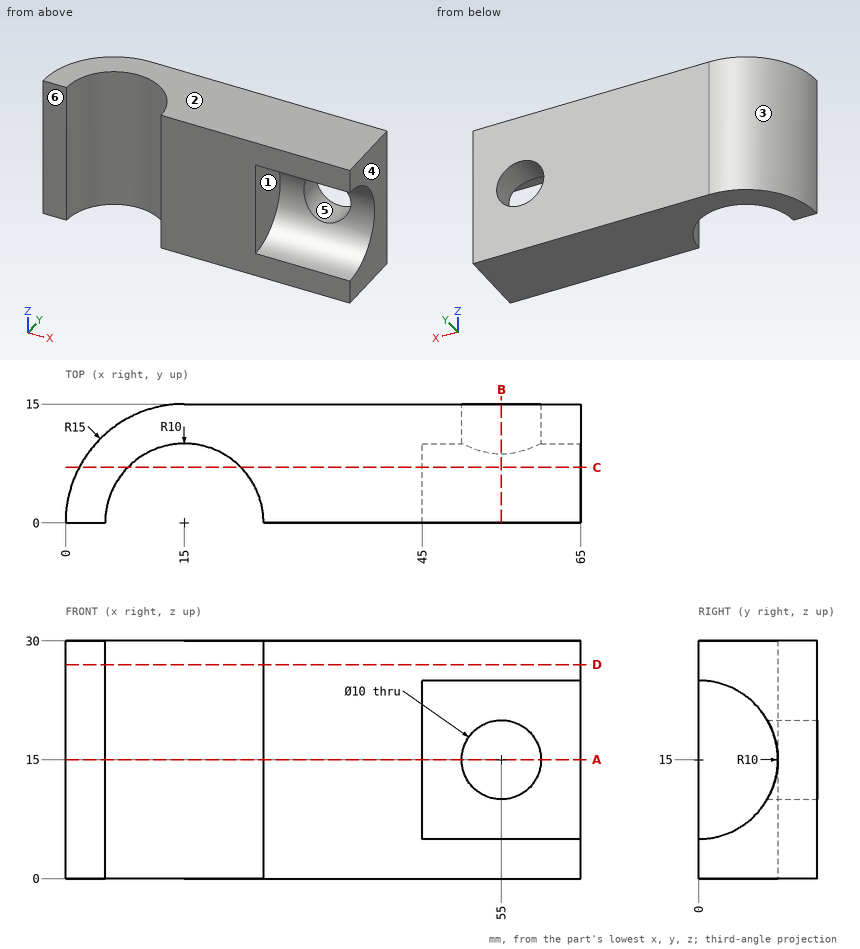
Could you check a few things on this drawing? It's one solid part, dimensions in mm from its lowest x, y, z. A direction names the side the tool comes from. Coordinates: 2 decimals unless noted, no trailing zeros. Order: outer loops, then holes, each group sorted by start corner. A loop starts at its lowest first (then second) coordinate and runs counter-clockwise, first axis right, second up.
1) Imagine slicing it at B-B on x = 55. List the corners of the cut face in (y, z) for me.
2) Imagine slicing it at D-D on z = 27. List the corners of the cut face in (x, y) for me, and give its area (3 significant figures).
3) We'd pull the mould along X, two halves only. Please class the marked faces 3, 4, 5 and 6: +X half, -X half, draft (parallel to the pull), parting line (faces both ways), or undercut.
4) Will these pins go through, and if not, where does the flat tip stop? pin 1 (5 mm diameter, centred on y = 5, z = 18.5, fed in from +X); pin 2 (1 mm diameter, centred on y = 11, z = 6, fed in from -X).
5) Imagine slicing it at A-A on z = 15. List the corners of the cut face in (x, y) for me.
6) Imagine slicing it at C-C on y = 7. List the corners of the cut face in (x, z) for me, and give its area (3 significant figures).
7) Which directions (+Z, -Z, +X, -X, +Y, -Y) give clear straight access to the entire face, cutting with the end or side of a thin tool? Please do the marked faces 1 and 2.
8) I need wall thicknesses on line 1 (Z direction, x = 55, y = 12.75); line 2 (X direction, y = 1, z = 27.5); line 3 (Z direction, x = 56, y = 1). Which ranges of each line are inside material? Lowest first, please.
Response values:
1. outline: (0, 0) - (15, 0) - (15, 10) - (8.66, 10) arc R10 cw to (0, 5) - close; (0, 25) arc R10 cw to (8.66, 20) - (15, 20) - (15, 30) - (0, 30) - close
2. outline: (0, 0) - (5, 0) arc R10 cw to (25, 0) - (65, 0) - (65, 15) - (15, 15) arc R15 ccw to start
2. area: 770 mm2
3. face 3: -X half
3. face 4: +X half
3. face 5: undercut
3. face 6: draft
4. pin 1: stops at x = 45
4. pin 2: stops at x = 4.29
5. outline: (0, 0) - (5, 0) arc R10 cw to (25, 0) - (45, 0) - (45, 10) - (50, 10) - (50, 15) - (15, 15) arc R15 ccw to start; (60, 10) - (65, 10) - (65, 15) - (60, 15) - close
6. outline: (1.73, 0) - (7.86, 0) - (7.86, 30) - (1.73, 30) - close; (22.14, 0) - (65, 0) - (65, 7.86) - (45, 7.86) - (45, 22.14) - (65, 22.14) - (65, 30) - (22.14, 30) - close
6. area: 1,180 mm2
7. face 1: +X, -Y
7. face 2: +Z, +X, -X, +Y, -Y
8. line 1: z = 0 to 10, 20 to 30
8. line 2: x = 0.03 to 5.05, 24.95 to 65
8. line 3: z = 0 to 5.05, 24.95 to 30
